Autodesk Inventor part; units mm, degrees
ref_plane "YZ Plane" through (0, 0, 0) normal (1, 0, 0) x (0, 1, 0)
ref_plane "XZ Plane" through (0, 0, 0) normal (0, 1, 0) x (-1, 0, 0)
ref_plane "XY Plane" through (0, 0, 0) normal (0, 0, 1) x (1, 0, 0)
sketch "Esquisse1" plane through (0, 0, 0) normal (0, 1, 0) x (-1, 0, 0)
  circle A0 centre (-28.5, 0) radius 3.5
  circle A1 centre (28.5, 0) radius 3.5
  line L0 (-35.5, 10) -> (35.5, 10)
  line L1 (35.5, 10) -> (35.5, -10)
  line L2 (35.5, -10) -> (-35.5, -10)
  line L3 (-35.5, -10) -> (-35.5, 10)
  line L4 (-28.5, 0) -> (28.5, 0)
  point P0 (0, 0)
  dimension "d0" = 7
  dimension "d1" = 7
  dimension "d2" = 28.5
  dimension "d3" = 28.5
  dimension "d4" = 20
  dimension "d5" = 10
  dimension "d6" = 7
  dimension "d7" = 7
extrude "Extrusion1" add sketch "Esquisse1" along normal blind 22
sketch "Esquisse2" plane through (0, 22, 0) normal (0, 1, 0) x (1, 0, 0)
  circle A0 centre (-28.5, 0) radius 3.5
  circle A1 centre (28.5, 0) radius 3.5
  line L0 (-23.5, 7.5) -> (23.5, 7.5)
  line L1 (23.5, 7.5) -> (23.5, -7.5)
  line L2 (23.5, -7.5) -> (-23.5, -7.5)
  line L3 (-23.5, -7.5) -> (-23.5, 7.5)
  point P0 (0, 0)
  dimension "d10" = 15
  dimension "d11" = 7.5
  dimension "d12" = 5
  dimension "d13" = 5
extrude "Extrusion2" cut sketch "Esquisse2" against normal through all contours L0 L1 L2 L3
sketch "Esquisse3" plane through (-35.5, 0, 10) normal (0, 0, 1) x (1, 0, 0)
  line L0 (71, 0) -> (0, 0)
  line L1 (71, 0) -> (71, 22)
  line L2 (0, 22) -> (71, 22)
  line L3 (0, 0) -> (0, 22)
  line L4 (14, 22) -> (57, 22)
  line L5 (57, 22) -> (57, 0)
  line L6 (57, 0) -> (14, 0)
  line L7 (14, 0) -> (14, 22)
  line L8 (14, 22) -> (22, 22)
  line L9 (22, 22) -> (22, 14)
  line L10 (22, 14) -> (14, 14)
  line L11 (14, 14) -> (14, 22)
  line L12 (57, 22) -> (49, 22)
  line L13 (49, 22) -> (49, 14)
  line L14 (49, 14) -> (57, 14)
  line L15 (57, 14) -> (57, 22)
  line L16 (14, 22) -> (22, 14)
  line L17 (22, 22) -> (14, 14)
  line L18 (49, 14) -> (57, 22)
  line L19 (49, 22) -> (57, 14)
  circle A0 centre (18, 18) radius 2
  circle A1 centre (53, 18) radius 2
  point P0 (35.5, 0)
  dimension "d16" = 14
  dimension "d17" = 14
  dimension "d18" = 8
  dimension "d19" = 8
  dimension "d20" = 8
  dimension "d21" = 8
  dimension "d22" = 4
  dimension "d23" = 4
sketch "Esquisse3 outline for Extrusion3" plane through (-35.5, 0, 10) normal (0, 0, 1) x (1, 0, 0)
  circle A0 centre (18, 18) radius 2
  circle A1 centre (53, 18) radius 2
extrude "Extrusion3" add sketch "Esquisse3 outline for Extrusion3" along normal through all both and the other way through all
sketch "Esquisse4" plane through (35.5, 0, 10) normal (1, 0, 0) x (0, 0, -1)
  line L0 (20, 0) -> (0, 0)
  line L1 (0, 22) -> (20, 22)
  line L2 (6.5, 22) -> (13.5, 22)
  line L3 (13.5, 22) -> (13.5, 0)
  line L4 (13.5, 0) -> (6.5, 0)
  line L5 (6.5, 0) -> (6.5, 22)
  circle A0 centre (5, 7.5) radius 1.5
  circle A1 centre (15, 7.5) radius 1.5
  line L6 (20, 0) -> (20, 22)
  line L7 (0, 0) -> (6.5, 0)
  line L8 (6.5, 0) -> (6.5, 15)
  line L9 (6.5, 15) -> (0, 15)
  line L10 (0, 15) -> (0, 0)
  line L11 (13.5, 0) -> (20, 0)
  line L12 (20, 0) -> (20, 15)
  line L13 (20, 15) -> (13.5, 15)
  line L14 (13.5, 15) -> (13.5, 0)
  line L15 (0, 0) -> (0, 22)
  line L16 (13.5, 7.5) -> (20, 7.5)
  line L17 (0, 7.5) -> (6.5, 7.5)
  point P0 (10, 0)
  dimension "d26" = 7
  dimension "d27" = 3.5
  dimension "d28" = 3
  dimension "d29" = 3
  dimension "d32" = 15
extrude "Extrusion4" cut sketch "Esquisse4" against normal through all contours L16 A1 | A1 L16 | L17 A0 | A0 L17
sketch "Esquisse5" plane through (-35.5, 0, 10) normal (0, 0, 1) x (1, 0, 0)
  line L0 (71, 0) -> (0, 0)
  line L1 (71, 0) -> (71, 22)
  line L2 (0, 22) -> (71, 22)
  line L3 (0, 0) -> (0, 22)
  line L4 (0, 0) -> (71, 0)
  line L5 (71, 0) -> (71, 11)
  line L6 (71, 11) -> (0, 11)
  line L7 (0, 11) -> (0, 0)
  point P0 (35.5, 0)
  dimension "d33" = 11
  dimension "d34" = 22
extrude "Extrusion5" cut sketch "Esquisse5" against normal through all both and the other way through all contours L6 L3 L2 L1
sketch "Esquisse6" plane through (-35.5, 11, 10) normal (0, 1, 0) x (1, 0, 0)
  line L0 (71, 0) -> (0, 0)
  line L1 (59, 2.5) -> (59, 17.5)
  line L2 (12, 2.5) -> (59, 2.5)
  line L3 (59, 2.5) -> (59, 0)
  line L4 (59, 0) -> (12, 0)
  line L5 (12, 0) -> (12, 2.5)
  line L6 (0, 0) -> (12, 0)
  line L7 (12, 0) -> (12, 2.5)
  line L8 (12, 2.5) -> (0, 2.5)
  line L9 (0, 2.5) -> (0, 0)
  line L10 (71, 0) -> (59, 0)
  line L11 (59, 0) -> (59, 2.5)
  line L12 (59, 2.5) -> (71, 2.5)
  line L13 (71, 2.5) -> (71, 0)
  point P0 (35.5, 10)
extrude "Extrusion6" add sketch "Esquisse6" along normal blind 11
sketch "Esquisse7" plane through (-35.5, 0, 10) normal (0, 0, 1) x (1, 0, 0)
  line L0 (0, 22) -> (71, 22)
  line L1 (35.5, 0) -> (35.5, 22)
  line L2 (35.5, 0) -> (35.5, -27)
  circle A0 centre (35.5, -27) radius 42.5
  point P0 (59, 22)
  point P1 (12, 22)
  dimension "d39" = 27
  dimension "d40" = 85
extrude "Extrusion7" cut sketch "Esquisse7" against normal blind 3
sketch "Esquisse8" plane through (-23.5, 11, 7.5) normal (0, 0, -1) x (-1, 0, 0)
  line L0 (12, 0) -> (-59, 0)
  line L1 (12, 0) -> (12, 11)
  line L2 (-59, 11) -> (12, 11)
  line L3 (-59, 0) -> (-59, 11)
  line L4 (-45, 11) -> (-2, 11)
  line L5 (-2, 11) -> (-2, 0)
  line L6 (-2, 0) -> (-45, 0)
  line L7 (-45, 0) -> (-45, 11)
  line L8 (-45, 11) -> (-37, 11)
  line L9 (-37, 11) -> (-37, 3)
  line L10 (-37, 3) -> (-45, 3)
  line L11 (-45, 3) -> (-45, 11)
  line L12 (-2, 11) -> (-10, 11)
  line L13 (-10, 11) -> (-10, 3)
  line L14 (-10, 3) -> (-2, 3)
  line L15 (-2, 3) -> (-2, 11)
  line L16 (-45, 11) -> (-37, 3)
  line L17 (-37, 11) -> (-45, 3)
  line L18 (-10, 3) -> (-2, 11)
  line L19 (-10, 11) -> (-2, 3)
  circle A0 centre (-41, 7) radius 2.5
  circle A1 centre (-6, 7) radius 2.5
  point P0 (-23.5, -11)
  point P1 (35.5, 0)
  dimension "d43" = 14
  dimension "d44" = 14
  dimension "d45" = 8
  dimension "d46" = 8
  dimension "d47" = 8
  dimension "d48" = 8
  dimension "d49" = 5
  dimension "d50" = 5
extrude "Extrusion8" cut sketch "Esquisse8" against normal through all contours A1 L18 L19 | L19 L18 A1 | L18 L19 A1 | A0 L16 L17 | L17 L16 A0 | A1 L19 L18 | A0 L17 L16 | L16 L17 A0
fillet "Congé1" radius 3 2 edges at (35.5, 5.5, -10) (-35.5, 5.5, -10)
equation "\"d5\" = 0.5 * d4"
equation "\"d17\" = d16"
equation "\"d44\" = d43"
properties part number "tendeur_base_low"
Could you check a few things on this model? Use its own coordinates, in mm. A direction names the side the tool comes from. Give positions to 0.01 mm unless a question says otherwise; leave off trailing zeros. Order: outer loops, then holes, each group sorted by start corner. A loop starts at its lowest first (then second) coordinate and runs counter-clockwise, first axis right, second up.
Q1. I'm going to push flat-ended pins straight in: P1, Ø4, axis at x = 8.5, y = 18.5, coming from the -Z side; P2, Ø1.8, axis at y = 7.5, z = 5, coming from the +X side; P3, Ø5.5, axis at x = 10.5, y = 4, coming from the +Z side; P4, Ø12, axis at x = -3, z = -2.5, coming from the +Y side. Where does each tip first touch, or does it pass through?
Q2. Suppose I cut it at D-D, the plane z = 5. Write out the boundary of the cut face in (x, y).
Q3. We'd pull the mould along X, two halves only. Please class faces 4 (the cylindrical face through (-16, 20, 9)), 5 (the flat face through (0, 22, 9)), 6 (the cylindrical face through (34.64, 5.58, -9.1)): +X half, -X half, draft (parallel to the pull), parting line (faces both ways), or undercut.
Q4. Suppose I cut it at B-B, the plane y = 18. Write out the boundary of the cut face in (x, z).
Q5. For faces 1 (the flat face through (-23.5, 6, 0)), 2 (the cylindrical face through (-34.6, 5.58, -9.14)), 3 (the flat face through (-27, 3, 7)), which set-ups out of +Z, -Z, +X, -X, +Y, -Y let a thin tool reach every point of the face, with its end or its side?
Q6. If I drill on line 1 along X through (y, z) = (18, 8.85); line 2 along X through (y, z) = (8.75, 0); line 3 along Y through (x, z) = (31, -5), over which ranges is the centre line in solid material (lowest first)?
Q7. Suppose I cut it at C-C, the plane x = -26.5. Write out the boundary of the cut face in (y, z), and give its area (3 significant figures).
Q8. Suppose I cut it at A-A, the plane z = 0. Write out the boundary of the cut face in (x, y), and give its area (3 significant figures).
Solution:
1. P1: stops at z = 7.5
1. P2: passes through
1. P3: stops at z = -7.5
1. P4: stops at y = 11
2. outline: (-35.5, 0) - (-23.5, 0) - (-23.5, 6) - (-35.5, 6) - close; (-35.5, 9) - (-23.5, 9) - (-23.5, 11) - (-35.5, 11) - close; (23.5, 0) - (35.5, 0) - (35.5, 6) - (23.5, 6) - close; (23.5, 9) - (35.5, 9) - (35.5, 11) - (23.5, 11) - close
3. face 4: undercut
3. face 5: draft
3. face 6: +X half
4. outline: (-35.5, 7.5) - (-20, 7.5) - (-20, 10) - (-35.5, 10) - close; (-15, 7.5) - (15, 7.5) - (15, 10) - (-15, 10) - close; (20, 7.5) - (35.5, 7.5) - (35.5, 10) - (20, 10) - close
5. face 1: +Y, -Y
5. face 2: -Z, -X, +Y, -Y
5. face 3: +Z, -Y
6. line 1: x = -35.5 to -20, -15 to 15, 20 to 35.5
6. line 2: x = -35.5 to -32, -25 to -23.5, 23.5 to 25, 32 to 35.5
6. line 3: y = 0 to 6, 9 to 11
7. outline: (0, -10) - (11, -10) - (11, -2.87) - (0, -2.87) - close; (0, 2.87) - (11, 2.87) - (11, 7.5) - (22, 7.5) - (22, 10) - (6.23, 10) - (6.23, 7) - (0, 7) - close; hole circle Ø3 at (7.5, -5); hole circle Ø3 at (7.5, 5)
7. area: 151 mm2
8. outline: (-35.5, 0) - (-32, 0) - (-32, 11) - (-35.5, 11) - close; (-25, 0) - (-23.5, 0) - (-23.5, 11) - (-25, 11) - close; (23.5, 0) - (25, 0) - (25, 11) - (23.5, 11) - close; (32, 0) - (35.5, 0) - (35.5, 11) - (32, 11) - close
8. area: 110 mm2
